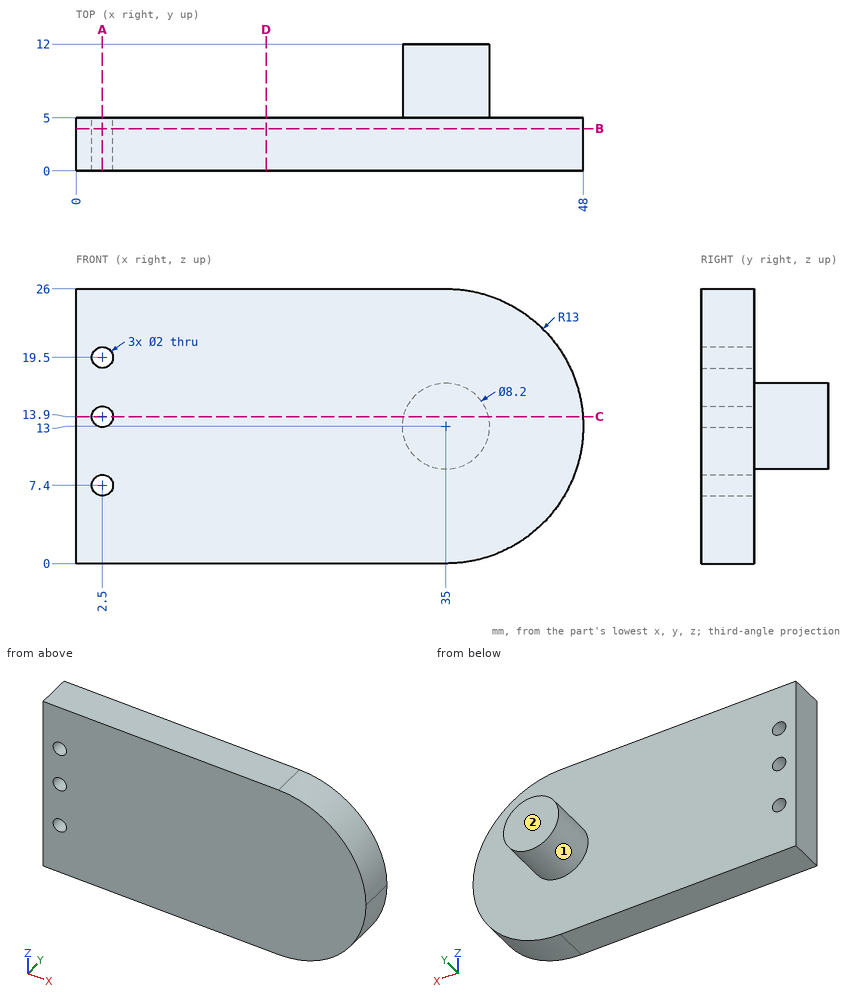
Answer from the drawing. Dimensions are ordinates in mm from the lowest x, y and z of the part. A direction names the side the tool comes from. Round coordinates to 2 decimals unless told otherwise and drop trailing zeros. Write each loop counter-clockwise with the first axis right and the second up, starting at its lowest first coordinate (ties: lowest second). Pieces come first, ordered by that corner, then holes.
1. Given pin 1 Ø12 at (x, z) = (25.5, 4.5) entering from +Y, flat-ended and moving along its own axis, determine where the tip first touches the part or whether it passes through.
2. The part is cut by section C-C, the plane z = 13.9. Determine the outline of the cut face in (x, y), then the cut area to 3 significant figures.
3. Which of the six approach directions +Z, -Z, +X, -X, +Y, -Y give full straight-line access (tool end or side, diameter ignored) to the marked faces 1 and 2?
4. The part is cut by section D-D, the plane x = 18. Determine the outline of the cut face in (y, z), then the cut area to 3 significant figures.
5. The part is cut by section B-B, the plane y = 4. Determine the outline of the cut face in (x, z).
6. The part is cut by section A-A, the plane x = 2.5. Determine the outline of the cut face in (y, z), then the cut area to 3 significant figures.
7. Straight lines are drawn through the part: L1, parallel to Z at x = 2.5, y = 3.8; L2, parallel to Z at x = 2, y = 4.75; L3, parallel to Y at x = 7, z = 18.75. For each, find the intervals that lie inside material, in ascending order.
Values:
1. pin 1: stops at y = 5
2. outline: (0, 0) - (1.5, 0) - (1.5, 5) - (0, 5) - close; (3.5, 0) - (47.97, 0) - (47.97, 5) - (39, 5) - (39, 12) - (31, 12) - (31, 5) - (3.5, 5) - close
2. area: 286 mm2
3. face 1: +Y
3. face 2: +Z, -Z, +X, -X, +Y
4. outline: (0, 0) - (5, 0) - (5, 26) - (0, 26) - close
4. area: 130 mm2
5. outline: (0, 0) - (35, 0) arc R13 ccw to (35, 26) - (0, 26) - close; hole circle Ø2 at (2.5, 7.4); hole circle Ø2 at (2.5, 13.9); hole circle Ø2 at (2.5, 19.5)
6. outline: (0, 0) - (5, 0) - (5, 6.4) - (0, 6.4) - close; (0, 8.4) - (5, 8.4) - (5, 12.9) - (0, 12.9) - close; (0, 14.9) - (5, 14.9) - (5, 18.5) - (0, 18.5) - close; (0, 20.5) - (5, 20.5) - (5, 26) - (0, 26) - close
6. area: 100 mm2
7. L1: z = 0 to 6.4, 8.4 to 12.9, 14.9 to 18.5, 20.5 to 26
7. L2: z = 0 to 6.53, 8.27 to 13.03, 14.77 to 18.63, 20.37 to 26
7. L3: y = 0 to 5
